from build123d import *

# Parameters (mm, degrees)
SKETCH1_R           = 5
BOSS_EXTRUDE1_DEPTH = 31.5
SKETCH2_R           = 1
CUT_EXTRUDE1_DEPTH  = 5
SKETCH3_R           = 7.5
BOSS_EXTRUDE2_DEPTH = 3


with BuildPart() as part:
    # Sketch1 → Boss-Extrude1 (new body)
    with BuildSketch(Plane.XY):
        Circle(SKETCH1_R)
    extrude(amount=BOSS_EXTRUDE1_DEPTH)

    # Sketch2 → Cut-Extrude1 (cut, symmetric)
    with BuildSketch(Plane(origin=(0, 0, 0), x_dir=(1, 0, 0), z_dir=(0, 1, 0))):
        with Locations(Location((0, -29, 0), (0, 0, 270))):
            Circle(SKETCH2_R)
    extrude(amount=CUT_EXTRUDE1_DEPTH, both=True, mode=Mode.SUBTRACT)

    # Sketch3 → Boss-Extrude2 (add)
    with BuildSketch(Plane(origin=(0, 0, 0), x_dir=(-1, 0, 0), z_dir=(0, 0, -1))):
        Circle(SKETCH3_R)
    extrude(amount=BOSS_EXTRUDE2_DEPTH)


solid = part.part
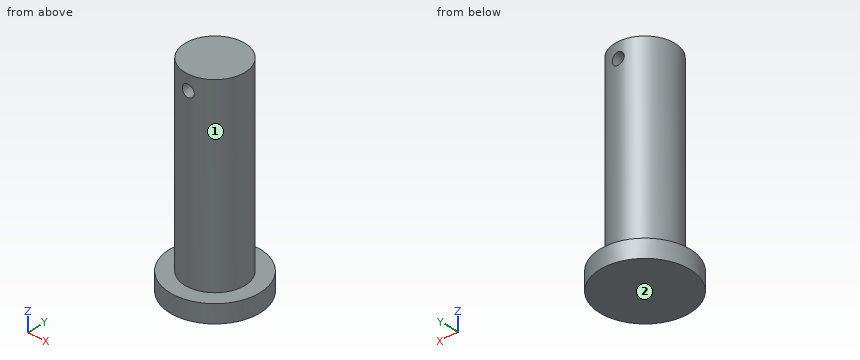
CAD build for the part. Positions are in the model's coordinates, mm. Face numbers are marked on the shaded views. A direction names the side the tool comes from. Give positions to 0.01 mm unless a question says otherwise; leave off trailing zeros. Loops run counter-clockwise (first coordinate to the right, second up) from the corner with the lowest first, then second, coordinate; pieces in that order, holes last. Notation, with made-up numbers: M 60.5,-5 L 74.5,-5 A28 ccw 74.5,20 Z; hole C -33.75,23.5 d9. An arc over 180 degrees is marked long. Answer in a Markdown table with one row per item. Add a question column.
Item 1: Probe probe 1 along Z at (x, y) = (0, 2.25); probe 2 along Y at (x, z) = (0, 5); probe 3 along Z at (x, y) = (5.5, 4.75). List the from-to ranges inside material, lowest first.
Item 2: Tool access for the marked faces 1 and 2: list every direction of +Z, -Z, +X, -X, +Y, -Y with a clear straight run to the whole face (end or side of a thin tool).
Item 3: Band-saw the part on D-D on z = 29. Give the cut face in (x, y).
Item 4: Drop flat-ended pins along their axis: P1, Ø3, axis at y = -4.5, z = 6, coming from the -X side; P2, Ø3, axis at y = -4.5, z = 25, coming from the +X side; P3, Ø2, axis at x = 5.5, z = 0.5, coming from the -Y side; P4, Ø1.8, axis at x = 0, z = 29, coming from the -Y side. Give the stop position or say it passes through.
Item 5: Band-saw the part on A-A on x = 0. Give the cut face in (y, z), then the cut area to 3 significant figures.
Item 6: Band-saw the part on C-C on x = -4. Give the cut face in (y, z).
Item 7: Band-saw the part on B-B on y = 0. Give the cut face in (x, z), then the cut area to 3 significant figures.
Reply:
| question | item | result |
|---|---|---|
| 1 | probe 1 | z = -3 to 28, 30 to 31.5 |
| 1 | probe 2 | y = -5 to 5 |
| 1 | probe 3 | z = -3 to 0 |
| 2 | face 1 | +Z |
| 2 | face 2 | -Z, +X, -X, +Y, -Y |
| 3 | outline | M -1,-4.9 L -1,4.9 A5 ccw Z; M 1,-4.9 A5 ccw 1,4.9 Z |
| 4 | P1 | stops at x = -4 |
| 4 | P2 | stops at x = 4 |
| 4 | P3 | stops at y = -5.9 |
| 4 | P4 | passes through |
| 5 | outline | M -7.5,-3 L 7.5,-3 L 7.5,0 L 5,0 L 5,28 L -5,28 L -5,0 L -7.5,0 Z; M -5,30 L 5,30 L 5,31.5 L -5,31.5 Z |
| 5 | area | 340 mm^2 |
| 6 | outline | M -6.34,-3 L 6.34,-3 L 6.34,0 L 3,0 L 3,31.5 L -3,31.5 L -3,0 L -6.34,0 Z |
| 7 | outline | M -7.5,-3 L 7.5,-3 L 7.5,0 L 5,0 L 5,31.5 L -5,31.5 L -5,0 L -7.5,0 Z; hole C 0,29 d2 |
| 7 | area | 357 mm^2 |
